The listing builds one solid part. Answer for the finished solid, in the listing's coordinates (mm). Face numbers are marked on the shaded views. A direction names the side the tool comes from. Give positions to 0.01 mm unless a question says otherwise; leave off trailing zeros. Write each loop counter-clockwise with the first axis right and the second up, starting at its lowest first coordinate (ties: lowest second). Pieces come first, ordered by that corner, then holes. Notation, with made-up numbers: (71.5, 11) - (122.5, 11) arc R20 ccw to (122.5, 21) - close; hole circle Ø4 at (26.5, 64.5). An arc over 180 degrees is marked (long way). Return JSON: item names as keys, results as strings.
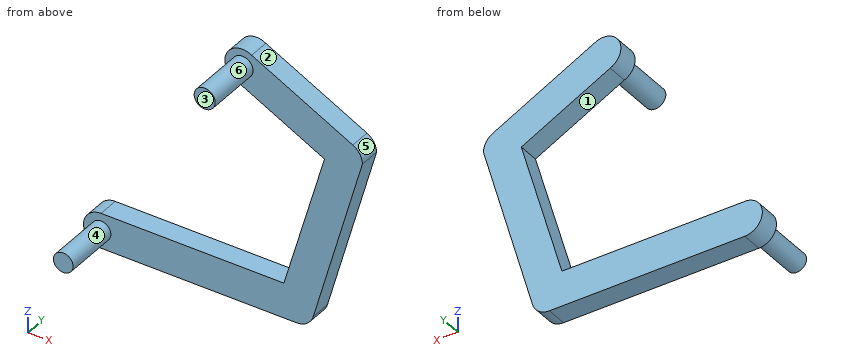
Autodesk Inventor part; units mm, degrees
ref_plane "YZ Plane" through (0, 0, 0) normal (1, 0, 0) x (0, 1, 0)
ref_plane "XZ Plane" through (0, 0, 0) normal (0, 1, 0) x (-1, 0, 0)
ref_plane "XY Plane" through (0, 0, 0) normal (0, 0, 1) x (1, 0, 0)
sketch "Sketch1" plane through (0, 0, 0) normal (0, 1, 0) x (-1, 0, 0)
  circle A0 centre (0, 0) radius 2.5
  circle A1 centre (-27.7848, -0.0003) radius 2.5
  circle A2 centre (-34.6699, 23.8458) radius 2.5
  circle A3 centre (-20.1174, 31.2789) radius 2.5
  line L0 (-32.1699, 23.8458) -> (-25.2848, -0.0003)
  line L1 (-37.1699, 23.8458) -> (-30.1893, -0.6845)
  line L2 (-27.9447, 2.4946) -> (-0.0005, 2.5)
  line L3 (-0.0005, -2.5) -> (-27.7848, -2.5003)
  line L4 (-19.1471, 28.9749) -> (-33.5318, 21.6199)
  arc A4 (-33.5318, 21.6199) -> (-35.8061, 26.0727) centre (-34.6699, 23.8458) ccw
  line L5 (-21.4171, 33.4145) -> (-35.8061, 26.0727)
  dimension "d0" = 5
  dimension "d1" = 5
  dimension "d2" = 5
  dimension "d3" = 5
extrude "Extrusion1" add sketch "Sketch1" along normal blind 3 contours A0 | A0 L3 A1 L0 L2 | L0 A1 L1 A2 L4 | A1 L0 | L4 A2 L0 | L0 A2 L5 A3 L4 | A1 L0 | A2 L1 | A3 picked at (-35.4421, 23.1763)
sketch "Sketch2" plane through (0, 0, 0) normal (0, -1, 0) x (1, 0, 0)
  circle A0 centre (0, 0) radius 1.4
  dimension "d6" = 2.8
extrude "Extrusion2" add sketch "Sketch2" along normal blind 8
thread "Thread3"
sketch "Sketch3" plane through (0, 3, 0) normal (0, 1, 0) x (1, 0, 0)
  point P0 (0, 0)
sketch "Sketch4" plane through (0, 0, 0) normal (0, -1, 0) x (1, 0, 0)
  arc A0 (21.4171, 33.4145) -> (19.1471, 28.9749) centre (20.1174, 31.2789) ccw
  circle A1 centre (20.1174, 31.2789) radius 1.5
  point P0 (0, 0)
  dimension "d15" = 3
extrude "Extrusion3" add sketch "Sketch4" along normal blind 8
thread "Thread4"
properties part number "Servo_Arm_Hook_new"
Item 1: A cutting plane is placed at A-A on z = 0. Determine the outline of the cut face in (x, y).
Answer below:
{"outline": "(-2.5, 0) - (-1.4, 0) - (-1.4, -8) - (1.4, -8) - (1.4, 0) - (30.38, 0) - (30.38, 3) - (-2.5, 3) - close"}
Item 2: Consider L1, parallel to Y at x = 19, z = 1; L2, parallel to Z at x = 8, y = 2.75; L3, parallel to Z at x = 20.5, y = 1.25. Determine where each line is inside the solid, lowest interval first.
Answer below:
{"L1": "y = 0 to 3", "L2": "z = -2.5 to 2.5", "L3": "z = -2.5 to 2.5, 28.28 to 33.75"}
Item 3: A cutting plane is placed at D-D on z = 21. Determine the outline of the cut face in (x, y).
Answer below:
{"outline": "(31.35, 0) - (36.36, 0) - (36.36, 3) - (31.35, 3) - close"}
Item 4: A cutting plane is placed at C-C on x = 6.5. Determine the outline of the cut face in (y, z).
Answer below:
{"outline": "(0, -2.5) - (3, -2.5) - (3, 2.5) - (0, 2.5) - close"}
Item 5: Flat-ended cylindrical pins translate along their axes: P1, Ø6, axis at y = 0.5, z = 27.5, coming from the +X side; P2, Ø4, axis at y = -0.5, z = 18, coming from the +X side; P3, Ø1.5, axis at x = 33, z = 11.5, coming from the -Y side. Find the tip coordinate at first contact, or state that the pin passes through.
Answer below:
{"P1": "stops at x = 37.08", "P2": "stops at x = 36.06", "P3": "stops at y = 0"}
Item 6: The mould has two halves that part along Z. Classify the marked faces 1, 2, 3 and 4: +Z half, -Z half, draft (parallel to the pull), parting line (faces both ways), or undercut.
Answer below:
{"face 1": "undercut", "face 2": "+Z half", "face 3": "draft", "face 4": "parting line"}
Item 7: For the marked faces 5 and 6, determine the directions among +Z, -Z, +X, -X, +Y, -Y from which every point of the face is accessible in a straight line to the end or side of a thin tool.
Answer below:
{"face 5": "+Z, +X, +Y, -Y", "face 6": "-Y"}
Item 8: A cutting plane is placed at B-B on y = -4.25. Determine the outline of the cut face in (x, z).
Answer below:
{"outline": "circle Ø2.8 at (0, 0); circle Ø3 at (20.12, 31.28)"}
